CAD build for the part. Positions are in the model's coordinates, mm. Give positions to 0.01 mm unless a question says otherwise; leave off trailing zeros. Loops run counter-clockwise (first coordinate to the right, second up) from the corner with the lowest first, then second, coordinate; pieces in that order, holes last. Notation, with made-up numbers: (84, 2.5) -> (137, 2.5) arc R33 ccw to (137, 31.5) -> close; hole circle Ø8 at (46.25, 1.5). An arc over 180 degrees is marked (long way). Use one line per item in the form item = value.
```python
from build123d import *

# Parameters (mm, degrees)
F0_W           = 69.8
F0_H           = 114.3
F0_W_2         = 33.5
F0_H_2         = 66.8
F1_DEPTH       = 6.4
F2_T           = -1
F3_R           = 2.4
F4_DEPTH       = 2
F5_DEPTH       = 2
F6_D           = 4
F6_CSINK_D     = 7
F6_CSINK_ANGLE = 90
F7_D           = 4
F7_CSINK_D     = 7
F7_CSINK_ANGLE = 90


# Not quite as in the source:
# - a feature names something its author has since deleted; it is built from what else it names


with BuildPart() as f1:
    # F0 (on Top) → F1 (new body)
    with BuildSketch(Plane.XY):
        with Locations((0, 8.7452211694)):
            Rectangle(F0_W, F0_H)
        with Locations((-0.15, 8.7452211694)):
            Rectangle(F0_W_2, F0_H_2, mode=Mode.SUBTRACT)
    extrude(amount=F1_DEPTH)

    # F2
    f2_openings = [f1.faces().sort_by_distance(p)[0] for p in [
        (0, 64.555948, 0),
    ]]
    offset(amount=F2_T, openings=f2_openings, kind=Kind.INTERSECTION)

    # F3 (on face) → F4 (join)
    with BuildSketch(Plane.XY.offset(6.4)):
        with Locations((30.9, -44.4047788306)):
            Circle(F3_R)
        with Locations((22.9, -44.4047788306)):
            Circle(F3_R)
        with Locations((14.9, -44.4047788306)):
            Circle(F3_R)
        with Locations((6.9, -44.2756973207)):
            Circle(F3_R)
        with Locations((-6.9, -44.4047788306)):
            Circle(F3_R)
        with Locations((-14.9, -44.4047788306)):
            Circle(F3_R)
        with Locations((-22.9, -44.4047788306)):
            Circle(F3_R)
        with Locations((-30.9, -44.4047788306)):
            Circle(F3_R)
        with Locations((-30.9, -36.4047788306)):
            Circle(F3_R)
        with Locations((-22.9, -36.4047788306)):
            Circle(F3_R)
        with Locations((-14.9, -36.4047788306)):
            Circle(F3_R)
        with Locations((-6.9, -36.2545885146)):
            Circle(F3_R)
        with Locations((6.9, -36.4047788306)):
            Circle(F3_R)
        with Locations((14.9, -36.4047788306)):
            Circle(F3_R)
        with Locations((22.9, -36.4047788306)):
            Circle(F3_R)
        with Locations((30.9, -36.4047788306)):
            Circle(F3_R)
        with Locations((30.9, -28.4047788306)):
            Circle(F3_R)
        with Locations((22.9, -28.4047788306)):
            Circle(F3_R)
        with Locations((14.9, -28.4047788306)):
            Circle(F3_R)
        with Locations((6.9, -28.4047788306)):
            Circle(F3_R)
        with Locations((0, -28.4047788306)):
            Circle(F3_R)
        with Locations((-6.9, -28.4047788306)):
            Circle(F3_R)
        with Locations((-14.9, -28.4047788306)):
            Circle(F3_R)
        with Locations((-22.9, -28.4047788306)):
            Circle(F3_R)
        with Locations((-30.9, -28.4047788306)):
            Circle(F3_R)
        with Locations((-30.9, -20.4047788306)):
            Circle(F3_R)
        with Locations((-22.9, -20.4047788306)):
            Circle(F3_R)
        with Locations((22.9, -20.4047788306)):
            Circle(F3_R)
        with Locations((30.9, -20.4047788306)):
            Circle(F3_R)
        with Locations((-30.9, -12.4047788306)):
            Circle(F3_R)
        with Locations((-30.9, -4.4047788306)):
            Circle(F3_R)
        with Locations((-30.9, 3.5952211694)):
            Circle(F3_R)
        with Locations((-30.9, 13.8952211694)):
            Circle(F3_R)
        with Locations((-30.9, 29.8952211694)):
            Circle(F3_R)
        with Locations((-30.9, 21.8952211694)):
            Circle(F3_R)
        with Locations((-30.9, 37.8952211694)):
            Circle(F3_R)
        with Locations((-22.9, 37.8952211694)):
            Circle(F3_R)
        with Locations((-22.9, 29.8952211694)):
            Circle(F3_R)
        with Locations((-22.9, 22.2151018679)):
            Circle(F3_R)
        with Locations((-22.9, 13.9829078689)):
            Circle(F3_R)
        with Locations((-22.9, 3.5952211694)):
            Circle(F3_R)
        with Locations((-22.9, -4.4047788306)):
            Circle(F3_R)
        with Locations((-22.9, -12.4047788306)):
            Circle(F3_R)
        with Locations((22.9, -12.4047788306)):
            Circle(F3_R)
        with Locations((22.9, -4.1701360606)):
            Circle(F3_R)
        with Locations((22.9, 3.6398950033)):
            Circle(F3_R)
        with Locations((23.0275392532, 13.9829078689)):
            Circle(F3_R)
        with Locations((22.9, 22.2151018679)):
            Circle(F3_R)
        with Locations((22.9, 29.8952211694)):
            Circle(F3_R)
        with Locations((22.9, 37.8952211694)):
            Circle(F3_R)
        with Locations((30.9, 37.8952211694)):
            Circle(F3_R)
        with Locations((30.9, 29.8952211694)):
            Circle(F3_R)
        with Locations((30.9, 21.8952211694)):
            Circle(F3_R)
        with Locations((30.9, 13.8952211694)):
            Circle(F3_R)
        with Locations((30.9, 3.5952211694)):
            Circle(F3_R)
        with Locations((30.9, -4.4047788306)):
            Circle(F3_R)
        with Locations((30.9, -12.4047788306)):
            Circle(F3_R)
        with Locations((-30.9, 61.8952211694)):
            Circle(F3_R)
        with Locations((-30.9, 53.8952211694)):
            Circle(F3_R)
        with Locations((-31.0094300658, 45.8952211694)):
            Circle(F3_R)
        with Locations((-22.9, 45.8952211694)):
            Circle(F3_R)
        with Locations((-22.9, 53.8952211694)):
            Circle(F3_R)
        with Locations((-22.9, 61.8952211694)):
            Circle(F3_R)
        with Locations((-14.9, 61.8952211694)):
            Circle(F3_R)
        with Locations((-14.9, 53.8952211694)):
            Circle(F3_R)
        with Locations((-14.9, 45.8562783897)):
            Circle(F3_R)
        with Locations((-6.9, 45.8952211694)):
            Circle(F3_R)
        with Locations((-6.9, 54.08847332)):
            Circle(F3_R)
        with Locations((-6.9, 61.8952211694)):
            Circle(F3_R)
        with Locations((6.9, 61.8952211694)):
            Circle(F3_R)
        with Locations((0, 45.8952211694)):
            Circle(F3_R)
        with Locations((6.9, 45.8952211694)):
            Circle(F3_R)
        with Locations((6.9, 53.8773909211)):
            Circle(F3_R)
        with Locations((14.9, 61.8952211694)):
            Circle(F3_R)
        with Locations((14.9, 53.8952211694)):
            Circle(F3_R)
        with Locations((14.9, 45.8952211694)):
            Circle(F3_R)
        with Locations((22.9, 53.8952211694)):
            Circle(F3_R)
        with Locations((22.9, 61.8952211694)):
            Circle(F3_R)
        with Locations((30.9, 61.8952211694)):
            Circle(F3_R)
        with Locations((30.9, 53.8952211694)):
            Circle(F3_R)
        with Locations((30.9, 45.8952211694)):
            Circle(F3_R)
    extrude(amount=F4_DEPTH)

    # F3 (on face) → F5 (join)
    with BuildSketch(Plane.XY.offset(6.4)):
        with Locations((22.9, 45.8952211694)):
            Circle(F3_R)
    extrude(amount=F5_DEPTH)

    # F6 (through all)
    with Locations(Plane.XY.offset(6.4)):
        with Locations((0, 57.1199804544)):
            CounterSinkHole(F6_D / 2, F6_CSINK_D / 2, counter_sink_angle=F6_CSINK_ANGLE)

    # F7 (through all)
    with Locations(Plane.XY.offset(6.4)):
        with Locations((0, -39.6666899323)):
            CounterSinkHole(F7_D / 2, F7_CSINK_D / 2, counter_sink_angle=F7_CSINK_ANGLE)


solid = f1.part
```
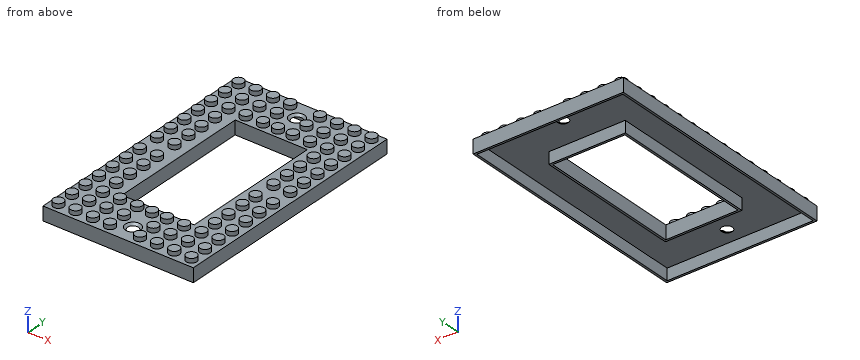
1. Drop a flat-ended pin along its axis: P1, Ø4, axis at y = 10, z = 7, coming from the -X side. Give the stop position or say it passes through.
Result sheet:
P1 = -34.9
2. Cut at A-A, the plane z = 4.25. Write the cut outline in (x, y), then the cut area to 3 significant figures.
Result sheet:
outline = (-34.9, -48.4) -> (34.9, -48.4) -> (34.9, 65.9) -> (-34.9, 65.9) -> close; (-17.9, -25.65) -> (17.6, -25.65) -> (17.6, 43.15) -> (-17.9, 43.15) -> close; hole (-33.9, -47.4) -> (33.9, -47.4) -> (33.9, 64.9) -> (-33.9, 64.9) -> close; hole (-16.9, -24.65) -> (16.6, -24.65) -> (16.6, 42.15) -> (-16.9, 42.15) -> close
area = 569 mm^2
3. Cut at B-B, the plane x = 0. State how many separate pieces and enclosed holes the cut face has, then the cut area to 3 significant figures.
Result sheet:
separate_pieces = 4
enclosed_holes = 0
area = 76.3 mm^2
4. Drill centre lines: line 1 (Y direction, x = 7.5, z = 4.5); line 2 (X direction, y = -8, z = 2); line 3 (X direction, y = 45, z = 3.75). Where is each one in solid material? Low to high.
Result sheet:
line_1 = -48.4 to -47.4, -25.65 to -24.65, 42.15 to 43.15, 64.9 to 65.9
line_2 = -34.9 to -33.9, -17.9 to -16.9, 16.6 to 17.6, 33.9 to 34.9
line_3 = -34.9 to -33.9, 33.9 to 34.9
